Work out the finished part from the listing and answer in its coordinate system (mm). Face numbers are marked on the shaded views. A direction names the side the tool comes from. Give positions to 0.01 mm unless a question says otherwise; leave off trailing zeros. Loops run counter-clockwise (first coordinate to the right, second up) from the corner with the lowest first, then second, coordinate; pieces in that order, holes last.
```python
from build123d import *

# Parameters (mm, degrees)
SKETCH_1_R            = 2.75
EXTRUDE_248_DEPTH     = 3
CUT_EXTRUDE_378_DEPTH = 1.3
SKETCH_3_R            = 1.5
EXTRUDE_479_DEPTH     = 30


with BuildPart() as part:
    # 草图1 → Extrude 248 (new body)
    with BuildSketch(Plane(origin=(0, 0, 0), x_dir=(1, 0, 0), z_dir=(0, 1, 0))):
        Circle(SKETCH_1_R)
    extrude(amount=EXTRUDE_248_DEPTH)

    # 草图2 → Cut-Extrude 378 (cut)
    with BuildSketch(Plane(origin=(0, 3, 0), x_dir=(1, 0, 0), z_dir=(0, 1, 0))):
        Polygon((1.443375673, 0), (0.721687836, 1.25), (-0.721687836, 1.25), (-1.443375673, 0), (-0.721687836, -1.25), (0.721687836, -1.25), align=None)
    extrude(amount=-CUT_EXTRUDE_378_DEPTH, mode=Mode.SUBTRACT)

    # 草图3 → Extrude 479 (add)
    with BuildSketch(Plane.XZ):
        Circle(SKETCH_3_R)
    extrude(amount=EXTRUDE_479_DEPTH)


solid = part.part
```
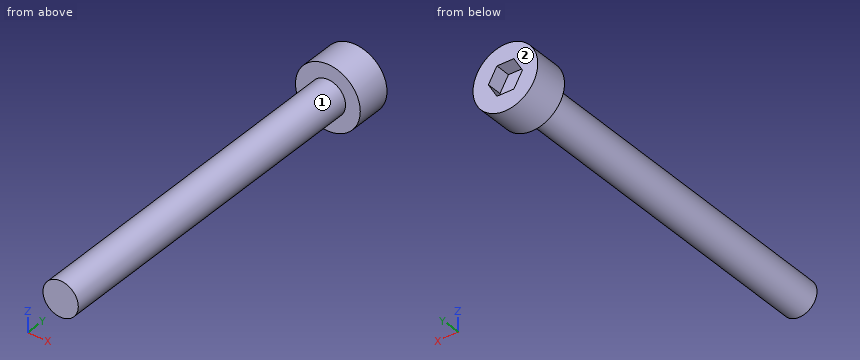
Q1. Given pin 1 (1 mm diameter, centred on y = -21, z = 0.5, fed in from -X); pin 2 (3 mm diameter, centred on x = 1.5, y = -14, fed in from +Z), each flat-ended and moving along its own axis, determine where each tip first touches the part or whether it passes through.
Q2. Which of the six approach directions +Z, -Z, +X, -X, +Y, -Y give full straight-line access (tool end or side, diameter ignored) to the marked faces 1 and 2?
Q3. Section D-D on x = -2.15 is taken. Give the vertices of the cut face in (y, z), plus the area to 3 significant figures.
Q4. Consider line 1 along Y through (x, z) = (1.25, -1.9); line 2 along Y through (x, z) = (-1, -0.3); line 3 along X through (y, z) = (-24, 0.05). Determine where each line is inside the solid, lowest interval first.
Q5. Section A-A on x = 0 is taken. Give the vertices of the cut face in (y, z), plus the area to 3 significant figures.
Q6. Section C-C on z = -2.05 is taken. Give the vertices of the cut face in (x, y), plus the area to 3 significant figures.
Q7. Section B-B on y = -17 is taken. Give the vertices of the cut face in (x, z), plus the area to 3 significant figures.
Check result:
1. pin 1: stops at x = -1.5
1. pin 2: stops at z = 1.5
2. face 1: -Y
2. face 2: +Z, -Z, +X, -X, +Y
3. outline: (0, -1.71) - (3, -1.71) - (3, 1.71) - (0, 1.71) - close
3. area: 10.3 mm2
4. line 1: y = 0 to 3
4. line 2: y = -30 to 1.7
4. line 3: x = -1.5 to 1.5
5. outline: (-30, -1.5) - (0, -1.5) - (0, -2.75) - (3, -2.75) - (3, -1.25) - (1.7, -1.25) - (1.7, 1.25) - (3, 1.25) - (3, 2.75) - (0, 2.75) - (0, 1.5) - (-30, 1.5) - close
5. area: 103 mm2
6. outline: (-1.83, 0) - (1.83, 0) - (1.83, 3) - (-1.83, 3) - close
6. area: 11.0 mm2
7. outline: circle Ø3 at (0, 0)
7. area: 7.07 mm2
